Could you check a few things on this model? Use its own coordinates, in mm. A direction names the side the tool comes from. Round coordinates to 2 decimals unless told otherwise and drop trailing zeros. Loops run counter-clockwise (first coordinate to the right, second up) from the corner with the lowest first, then second, coordinate; pieces in that order, holes last. Notation, with made-up numbers: (-18, 35) -> (0, 35) arc R27 cw to (0, 72) -> close; hole circle Ø7 at (7.25, 59.5). An arc over 180 degrees is marked (long way). One line per item, written item: value.
```python
from build123d import *

# Parameters (mm, degrees)
F1_DEPTH       = 6
F2_R           = 4
F3_R           = 8
F4_R           = 11
F5_R           = 1.99999
F7_D           = 3
F7_CSINK_D     = 5
F7_CSINK_ANGLE = 90


# Not quite as in the source:
# - a fillet or chamfer is up to 0.001 mm smaller than in the source, because OpenCascade refuses the exact size


with BuildPart() as f1:
    # F0 (on Front) → F1 (new body)
    with BuildSketch(Plane.XZ):
        Polygon((0, 0), (0, 30), (7, 30), (7, 34), (-4, 34), (-4, -4), (16, -4), (16, 26), (36, 26), (36, 38), (10, 38), (10, 0), align=None)
    extrude(amount=F1_DEPTH)

    # F2
    f2_edges = [f1.edges().sort_by_distance(p)[0] for p in [
        (10, -3, 0),
        (0, -3, 0),
        (0, -3, 30),
    ]]
    fillet(f2_edges, radius=F2_R)

    # F3
    f3_edges = [f1.edges().sort_by_distance(p)[0] for p in [
        (-4, -3, 34),
        (-4, -3, -4),
    ]]
    fillet(f3_edges, radius=F3_R)

    # F4
    f4_edges = [f1.edges().sort_by_distance(p)[0] for p in [
        (16, -3, -4),
    ]]
    fillet(f4_edges, radius=F4_R)

    # F5 (radius 2 in the source; OpenCascade refuses exactly that, so slightly less here)
    f5_edges = [f1.edges().sort_by_distance(p)[0] for p in [
        (7, -3, 34),
        (7, -3, 30),
    ]]
    fillet(f5_edges, radius=F5_R)

    # F7 (through all)
    with Locations(Plane(origin=(0, 0, 26), x_dir=(1, 0, 0), z_dir=(0, 0, -1))):
        with Locations((20, 3.0815127769), (31.9998442765, 3.0203789876)):
            CounterSinkHole(F7_D / 2, F7_CSINK_D / 2, counter_sink_angle=F7_CSINK_ANGLE)


solid = f1.part
```
(1) On a 3-axis mill with a long thin cutter (end or side, diameter ignored), from which of +Z, -Z, +X, -X, +Y, -Y can I reach the whole of each face in a straight line? I mean faces 1 (the face through (1.141, -3.042, 28.797)), 2 (the face through (36, -3, 32)), 3 (the face through (10, -3, 21)). Say none if no direction works.
Results below:
face 1: +Y, -Y
face 2: +Z, -Z, +X, +Y, -Y
face 3: +Z, +Y, -Y
(2) Imagine slicing it at A-A on x = 20. Write out the boundary of the cut face in (y, z).
Results below:
outline: (-6, 26) -> (-5.58, 26) -> (-4.58, 27) -> (-4.58, 38) -> (-6, 38) -> close; (-1.58, 27) -> (-0.58, 26) -> (0, 26) -> (0, 38) -> (-1.58, 38) -> close
(3) Please list where these lines run through material, in increasing order: L1, parallel to X at y = -4.4, z = 11; L2, parallel to Z at x = 17, y = -3.75; L3, parallel to Z at x = 1, y = -5.
Results below:
L1: x = -4 to 0, 10 to 16
L2: z = 26 to 38
L3: z = -3.42 to 1.35, 28.65 to 33.42
(4) We'd pull the mould along Y, two halves only. Please class faces 4 (the face through (4.5, -3, 34)), 5 (the face through (21.5, -3.1, 32.6)): +Y half, -Y half, draft (parallel to the pull), parting line (faces both ways), or undercut.
Results below:
face 4: draft
face 5: undercut
(5) Imagine slicing it at C-C on x = 4.5. Write out the boundary of the cut face in (y, z).
Results below:
outline: (-6, -4) -> (0, -4) -> (0, 0) -> (-6, 0) -> close; (-6, 30) -> (0, 30) -> (0, 34) -> (-6, 34) -> close
(6) Imagine slicing it at D-D on y = -2.2. Give the number of separate pieces and of enclosed holes in the cut face, then the cut area to 3 significant figures.
Results below:
separate pieces: 3
enclosed holes: 0
area: 606 mm²
(7) For pin 1 Ø3 at (y, z) = (-1.5, 12.5) entering from +X; pin 2 Ø1.8 at (x, y) = (22.5, -1.5) entering from -Z; pin 3 Ø3 at (y, z) = (-3.5, 26.5) entering from -X; pin 4 Ø2 at (x, y) = (5, -4.5) entering from +Z, each with a flat end and sliding along its axis, tell me the tip position at first contact or that it passes through.
Results below:
pin 1: stops at x = 16
pin 2: stops at z = 26
pin 3: stops at x = -4
pin 4: stops at z = 34
(8) Imagine slicing it at B-B on z = 21.5. Write out the boundary of the cut face in (x, y), then the cut area to 3 significant figures.
Results below:
outline: (-4, -6) -> (0, -6) -> (0, 0) -> (-4, 0) -> close; (10, -6) -> (16, -6) -> (16, 0) -> (10, 0) -> close
area: 60.0 mm²
